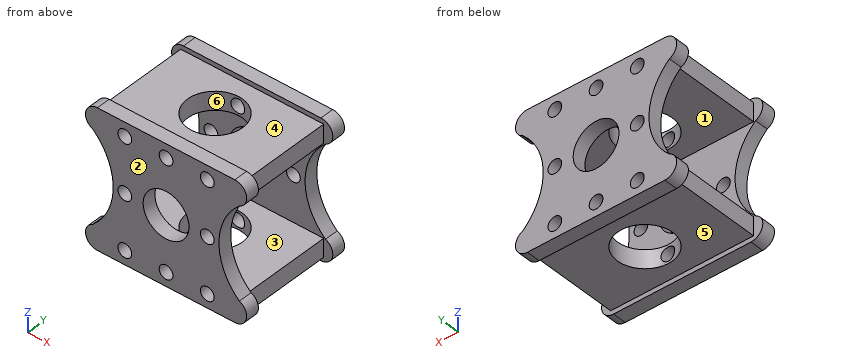
```python
from build123d import *

# Parameters (mm, degrees)
ESQUISSE1_R                  = 5
ESQUISSE1_R_2                = 1.5
BOSS_EXTRU_1_DEPTH           = 25
ESQUISSE2_W                  = 20
ESQUISSE2_H                  = 19
ESQUISSE2_W_2                = 4.56072091
ESQUISSE2_W_3                = 3.825642854
ENL_V_MAT_EXTRU_1_DEPTH      = 25
ENL_V_MAT_EXTRU_1_DEPTH_BACK = 25
ESQUISSE3_R                  = 6
ESQUISSE3_W                  = 8.37073205
ESQUISSE3_H                  = 19
ESQUISSE3_W_2                = 9.375022173
ENL_V_MAT_EXTRU_2_DEPTH      = 30


with BuildPart() as part:
    # Esquisse1 → Boss.-Extru.1 (new body)
    with BuildSketch(Plane(origin=(0, 0, 0), x_dir=(1, 0, 0), z_dir=(0, 1, 0))):
        with BuildLine():
            Line((-15, 15), (15, 15))
            ThreePointArc((15, 15), (17.549509757, 12.909901951), (16, 10))
            ThreePointArc((16, 10), (11.546375953, 0), (16, -10))
            ThreePointArc((16, -10), (17.549509757, -12.909901951), (15, -15))
            Line((15, -15), (-15, -15))
            ThreePointArc((-15, -15), (-17.549509757, -12.909901951), (-16, -10))
            ThreePointArc((-16, -10), (-11.546375953, 0), (-16, 10))
            ThreePointArc((-16, 10), (-17.549509757, 12.909901951), (-15, 15))
        make_face()
        Circle(ESQUISSE1_R, mode=Mode.SUBTRACT)
        with Locations((9, 0)):
            Circle(ESQUISSE1_R_2, mode=Mode.SUBTRACT)
        with Locations((-9, 0)):
            Circle(ESQUISSE1_R_2, mode=Mode.SUBTRACT)
        with Locations((-9, 12)):
            Circle(ESQUISSE1_R_2, mode=Mode.SUBTRACT)
        with Locations((9, 12)):
            Circle(ESQUISSE1_R_2, mode=Mode.SUBTRACT)
        with Locations((-9, -12)):
            Circle(ESQUISSE1_R_2, mode=Mode.SUBTRACT)
        with Locations((9, -12)):
            Circle(ESQUISSE1_R_2, mode=Mode.SUBTRACT)
        with Locations((0, -12)):
            Circle(ESQUISSE1_R_2, mode=Mode.SUBTRACT)
        with Locations((0, 12)):
            Circle(ESQUISSE1_R_2, mode=Mode.SUBTRACT)
    extrude(amount=BOSS_EXTRU_1_DEPTH)

    # Esquisse2 → Enl_v. mat.-Extru.1 (cut, two sides)
    with BuildSketch(Plane(origin=(0, 0, 0), x_dir=(0, 0, -1), z_dir=(1, 0, 0))) as enl_v_mat_extru_1_sk:
        with Locations((0, 12.5)):
            Rectangle(ESQUISSE2_W, ESQUISSE2_H)
        with Locations((16.280360455, 12.5)):
            Rectangle(ESQUISSE2_W_2, ESQUISSE2_H)
        with Locations((-15.912821427, 12.5)):
            Rectangle(ESQUISSE2_W_3, ESQUISSE2_H)
    extrude(amount=ENL_V_MAT_EXTRU_1_DEPTH, mode=Mode.SUBTRACT)
    extrude(enl_v_mat_extru_1_sk.sketch, amount=-ENL_V_MAT_EXTRU_1_DEPTH_BACK, mode=Mode.SUBTRACT)

    # Esquisse3 → Enl_v. mat.-Extru.2 (cut)
    with BuildSketch(Plane.XY.offset(14)):
        with Locations((0, 12.5)):
            Circle(ESQUISSE3_R)
        with Locations((-19.785366025, 12.5)):
            Rectangle(ESQUISSE3_W, ESQUISSE3_H)
        with Locations((20.287511087, 12.5)):
            Rectangle(ESQUISSE3_W_2, ESQUISSE3_H)
    extrude(amount=-ENL_V_MAT_EXTRU_2_DEPTH, mode=Mode.SUBTRACT)


solid = part.part
```
Part model, mm, in its own coordinate system. Face numbers are marked on the shaded views. A direction names the side the tool comes from. Round coordinates to 2 decimals unless told otherwise and drop trailing zeros. Order: outer loops, then holes, each group sorted by start corner. A loop starts at its lowest first (then second) coordinate and runs counter-clockwise, first axis right, second up. Notation, with made-up numbers: M -1,-24 L 27,-24 A26 cw 27,-2 Z; hole C 43.25,8.5 d11. An arc over 180 degrees is marked long. Put each result on its own line as item: value. Start each with the question number.
1. Drill centre lines: probe 1 along Z at (x, y) = (0, 4.5); probe 2 along X at (y, z) = (2.35, 0); probe 3 along Z at (x, y) = (-9, 1.4). Where is each one in solid material? Low to high. Write a range as [from, to].
2. Tool access for the marked faces 5 and 6: list every direction of +Z, -Z, +X, -X, +Y, -Y with a clear straight run to the whole face (end or side of a thin tool).
3. Slice it at B-B on z = 0. State how many separate pieces and enclosed holes the cut face has, then the cut area to 3 significant figures.
4. Drop flat-ended pins along their axis: pin 1 (1.8 mm diameter, centred on x = 9, z = 0, fed in from +Y); pin 2 (2 mm diameter, centred on y = 9, z = -12, fed in from +X); pin 3 (1.5 mm diameter, centred on x = -14, y = 18.5, fed in from -Z); pin 4 (6 mm diameter, centred on x = -11, y = 13, fed in from +Z). Give the stop position or say it passes through.
5. Slice it at A-A on y = 12.5. List the corners of the cut face in (x, z).
6. Two-plate mould, pull along Z, no slides. Class the marked faces 1, 2, 3 and 4: +Z half, -Z half, draft (parallel to the pull), parting line (faces both ways), or undercut.
7. Slice it at D-D on z = 6. List the corners of the cut face in (x, y), then the cut area to 3 significant figures.
Findings:
1. probe 1: [-14, -13.5], [-10.5, -10], [10, 10.5], [13.5, 14]
1. probe 2: [-11.55, -10.5], [-7.5, -5], [5, 7.5], [10.5, 11.55]
1. probe 3: [-15, -13.5], [-10.5, -1.5], [1.5, 10.5], [13.5, 15]
2. face 5: -Z, +X, -X
2. face 6: +Z, -Z
3. separate pieces: 8
3. enclosed holes: 0
3. area: 42.6 mm2
4. pin 1: through
4. pin 2: x = 15.6
4. pin 3: z = -14
4. pin 4: z = 14
5. outline: M -15.6,-14 L -6,-14 L -6,-10 L -15.6,-10 Z; M -15.6,10 L -6,10 L -6,14 L -15.6,14 Z; M 6,-14 L 15.6,-14 L 15.6,-10 L 6,-10 Z; M 6,10 L 15.6,10 L 15.6,14 L 6,14 Z; hole C -9,-12 d3; hole C -9,12 d3; hole C 9,-12 d3; hole C 9,12 d3
6. face 1: undercut
6. face 2: draft
6. face 3: undercut
6. face 4: +Z half
7. outline: M -12.96,0 L 12.96,0 L 12.96,3 L -12.96,3 Z; M -12.96,22 L 12.96,22 L 12.96,25 L -12.96,25 Z
7. area: 156 mm2
